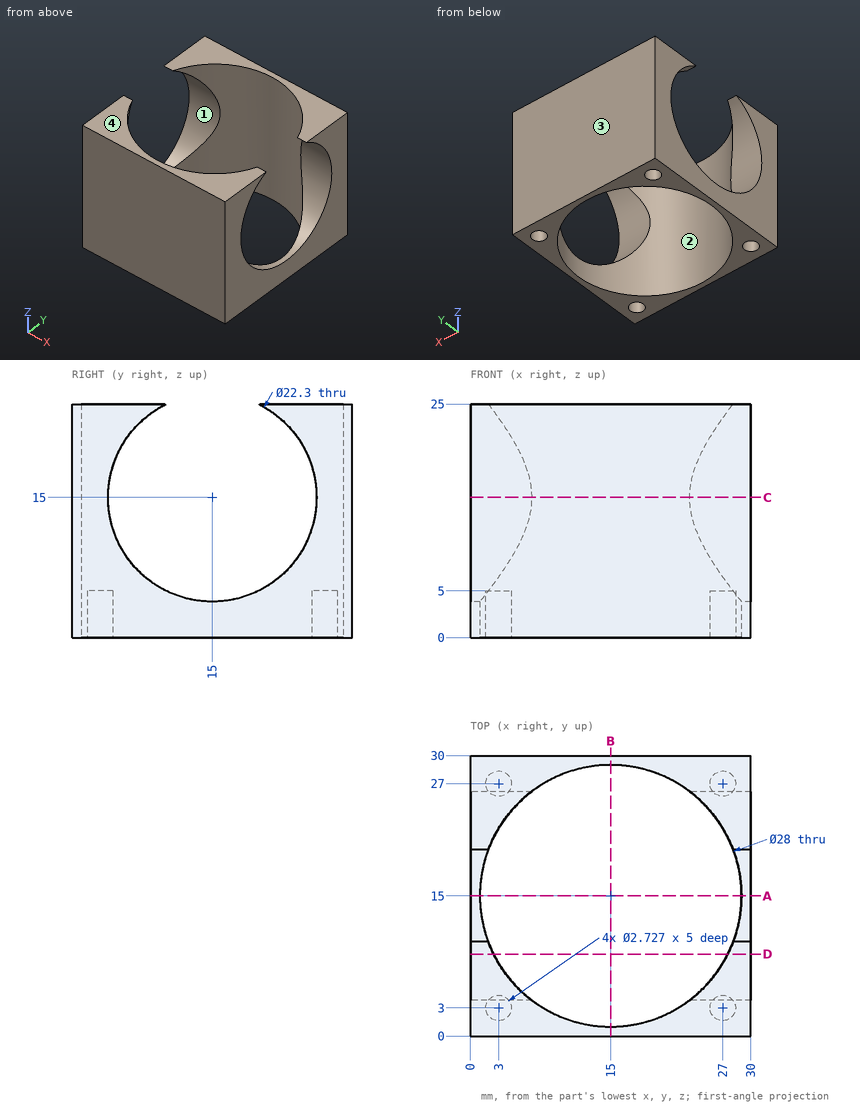
Verification items for this drawing (mm, ordinates from the low corner). Round coordinates to 2 decimals unless told otherwise and drop trailing zeros. Write each loop counter-clockwise with the first axis right and the second up, starting at its lowest first coordinate (ties: lowest second). Pieces come first, ordered by that corner, then holes. Notation, with made-up numbers: (-24.75, 30.5) - (16.25, 30.5) arc R19 ccw to (16.25, 41.5) - close; hole circle Ø10 at (-11, 1.25). An arc over 180 degrees is marked (long way). Answer as a JSON object with one key per item and string values. Group by question number.
Q1. Section check A-A, the plane y = 15. Enter the section's corners in (x, z).
Q2. Mould release check, pull along Y, two halves, no side actions. Record for the marked faces 1, 2, 3 and 4: released by +Y, released by -Y, zero draft, split by the parting line, or undercut.
Q3. Thickness scan on line 1 (Y direction, x = 27.5, z = 15); line 2 (Y direction, x = 3, z = 2.15) (1 decimal); line 3 (Y direction, x = 2, z = 22.25). Record the ranges inside material, lowest first.
Q4. Section check C-C, the plane z = 15. Enter the section's corners in (x, y), plus the area to 3 significant figures.
Q5. Section check D-D, the plane y = 8.75. Enter the section's corners in (x, z).
Q6. Section check B-B, the plane x = 15. Enter the section's corners in (y, z).
Q7. Go/stop test with flat-tipped pins: pin 1 Ø5 at (y, z) = (21, 13.5) entering from -X; pin 2 Ø0.8 at (x, y) = (3.5, 27.5) entering from -Z. Record where each tip stops, or that it passes through.
Found:
{
 "1": {"outline": "(0, 0) - (1, 0) - (1, 3.85) - (0, 3.85) - close; (29, 0) - (30, 0) - (30, 3.85) - (29, 3.85) - close"},
 "2": {"face 1": "undercut", "face 2": "undercut", "face 3": "released by +Y", "face 4": "zero draft"},
 "3": {"line 1": "y = 0 to 3.85, 26.15 to 30", "line 2": "y = 0 to 1.6, 4.4 to 7.8, 22.2 to 25.6, 28.4 to 30", "line 3": "y = 0 to 6.53, 23.47 to 30"},
 "4": {"outline": "(0, 0) - (30, 0) - (30, 3.85) - (23.47, 3.85) arc R14 cw to (6.53, 3.85) - (0, 3.85) - close; (0, 26.15) - (6.53, 26.15) arc R14 cw to (23.47, 26.15) - (30, 26.15) - (30, 30) - (0, 30) - close", "area": "165 mm^2"},
 "5": {"outline": "(0, 0) - (2.47, 0) - (2.47, 5.77) - (0, 5.77) - close; (0, 24.23) - (2.47, 24.23) - (2.47, 25) - (0, 25) - close; (27.53, 0) - (30, 0) - (30, 5.77) - (27.53, 5.77) - close; (27.53, 24.23) - (30, 24.23) - (30, 25) - (27.53, 25) - close"},
 "6": {"outline": "(0, 0) - (1, 0) - (1, 25) - (0, 25) - close; (29, 0) - (30, 0) - (30, 25) - (29, 25) - close"},
 "7": {"pin 1": "passes through", "pin 2": "stops at z = 5"}
}
